```python
from build123d import *

# Parameters (mm, degrees)
SKETCH_1_W                   = 36
SKETCH_1_H                   = 18.5
EXTRUDE_1_DEPTH              = 8
HOLE_WIZARD_M2_1_D           = 2.4
HOLE_WIZARD_M2_1_CBORE_D     = 4.4
HOLE_WIZARD_M2_1_CBORE_DEPTH = 3.5
SKETCH_8_W                   = 60
SKETCH_8_H                   = 30
EXTRUDE_2_DEPTH              = 10
EXTRUDE_3_DEPTH              = 2.5


with BuildPart() as part:
    # 草图1 → 凸台-拉伸1 (new body)
    with BuildSketch(Plane(origin=(0, 0, 0), x_dir=(1, 0, 0), z_dir=(0, 1, 0))):
        with Locations((-18, 0)):
            Rectangle(SKETCH_1_W, SKETCH_1_H)
        Polygon((-6.8, 6.25), (-29.2, 6.25), (-33, 6.25), (-33, -6.25), (-29.2, -6.25), (-6.8, -6.25), align=None, mode=Mode.SUBTRACT)
    extrude(amount=EXTRUDE_1_DEPTH)

    # M2 凹头盖螺钉的柱形沉头孔1 (through all)
    with Locations(Plane(origin=(-4.15, 8, 0), x_dir=(0, 0, 1), z_dir=(0, 1, 0))):
        with Locations((0, 0)):
            CounterBoreHole(HOLE_WIZARD_M2_1_D / 2, HOLE_WIZARD_M2_1_CBORE_D / 2, HOLE_WIZARD_M2_1_CBORE_DEPTH)

    # 草图4 → 放样1 section 0
    with BuildSketch(Plane(origin=(0, 0, 0), x_dir=(0, 0, -1), z_dir=(1, 0, 0))):
        with BuildLine():
            Line((9.25, 8), (-9.25, 8))
            Line((-9.25, 8), (-9.25, 0))
            Line((-9.25, 0), (9.25, 0))
            Line((9.25, 0), (9.25, 8))
        make_face()
    # 草图5 → 放样1 section 1
    with BuildSketch(Plane(origin=(60, 0, 0), x_dir=(0, 0, -1), z_dir=(1, 0, 0))):
        with BuildLine():
            Line((-2.5, 8), (2.5, 8))
            Line((2.5, 8), (2.5, 0))
            Line((2.5, 0), (-2.5, 0))
            Line((-2.5, 0), (-2.5, 8))
        make_face()
    loft()

    # 草图8 → 凸台-拉伸2 (add)
    with BuildSketch(Plane(origin=(60, 0, 0), x_dir=(0, 0, -1), z_dir=(1, 0, 0))):
        with Locations((0, 15)):
            Rectangle(SKETCH_8_W, SKETCH_8_H)
    extrude(amount=-EXTRUDE_2_DEPTH)

    # 草图11 → 凸台-拉伸3 (add, symmetric)
    with BuildSketch(Plane.XY):
        Polygon((50, 28), (20, 8), (50, 8), align=None)
    extrude(amount=EXTRUDE_3_DEPTH, both=True)


solid = part.part
```
The model under review builds one solid part; all positions refer to its coordinate system, in mm. A direction names the side the tool comes from. Coordinates: 2 decimals unless noted, no trailing zeros. Loops run counter-clockwise (first coordinate to the right, second up) from the corner with the lowest first, then second, coordinate; pieces in that order, holes last. Notation, with made-up numbers: (-28, -19) -> (1, -19) arc R18 cw to (1, 5) -> close; hole circle Ø1 at (-17.75, 54.25). An arc over 180 degrees is marked (long way). Answer as CSV lines item,"result".
Item 1: Take a section at A-A, the plane x = -4.15. State the section outline as (y, z) points, and give its area (3 significant figures).
Results below:
outline,"(0, -9.25) -> (8, -9.25) -> (8, -2.2) -> (4.5, -2.2) -> (4.5, -1.2) -> (0, -1.2) -> close; (0, 1.2) -> (4.5, 1.2) -> (4.5, 2.2) -> (8, 2.2) -> (8, 9.25) -> (0, 9.25) -> close"
area,"122 mm2"
Item 2: Take a section at C-C, the plane y = 18.5. State the section outline as (x, z) points, and give its area (3 significant figures).
Results below:
outline,"(35.75, -2.5) -> (50, -2.5) -> (50, -30) -> (60, -30) -> (60, 30) -> (50, 30) -> (50, 2.5) -> (35.75, 2.5) -> close"
area,"671 mm2"
Item 3: Take a section at D-D, the plane z = 11. State the section outline as (x, y) points.
Results below:
outline,"(50, 0) -> (60, 0) -> (60, 30) -> (50, 30) -> close"
Item 4: Insertion check: pin 1 (4 mm diameter, centred on x = -4.15, z = 0, fed in from +Y); pin 2 (6 mm diameter, centred on x = 12.5, y = 6, fed in from -Z); pin 3 (6.5 mm diameter, centred on x = -17, y = 6, fed in from +Z); pin 4 (5 mm diameter, centred on x = -22.5, z = 3, fed in from +Y). Each pin has a flat end and moves straight along its axis. Give the tip position at first contact, or say it passes through.
Results below:
pin 1,"stops at y = 4.5"
pin 2,"stops at z = -8.18"
pin 3,"stops at z = 9.25"
pin 4,"passes through"
Item 5: Draft analysis for pull direction X (two halves, no side actions). For faces 1 (the cylindrical face through (-4.1, 6.3, -2.2)), 2 (the flat face through (55, 15, -30)), 3 (the flat face through (-36, 4, 0)), state which applies: +X half, -X half, draft (parallel to the pull), parting line (faces both ways), or undercut.
Results below:
face 1,"undercut"
face 2,"draft"
face 3,"-X half"
Item 6: For L1, parallel to X at y = 3, z = 0; L2, parallel to X at y = 6, z = 0; L3, parallel to Z at x = -4, y = 2, list the stretches that pass through material, from the lowest coordinate up.
Results below:
L1,"x = -36 to -33, -6.8 to -5.35, -2.95 to 60"
L2,"x = -36 to -33, -6.8 to -6.35, -1.95 to 60"
L3,"z = -9.25 to -1.19, 1.19 to 9.25"
Item 7: Take a section at B-B, the plane z = 0. State the section outline as (x, y) points.
Results below:
outline,"(-36, 0) -> (-33, 0) -> (-33, 8) -> (-36, 8) -> close; (-6.8, 0) -> (-5.35, 0) -> (-5.35, 4.5) -> (-6.35, 4.5) -> (-6.35, 8) -> (-6.8, 8) -> close; (-2.95, 0) -> (60, 0) -> (60, 30) -> (50, 30) -> (50, 28) -> (20, 8) -> (-1.95, 8) -> (-1.95, 4.5) -> (-2.95, 4.5) -> close"
Item 8: Machinability: for faces 4 (the flat face through (41, 14, 2.5)), 5 (the flat face through (25.35, 4.06, 6.4)), 6 (the flat face through (-4.1, 4.5, 1.4)), 7 (the flat face through (25.35, 3.94, -6.4)), 8 (the flat face through (-20, 4, 6.25)), which of the approach directions +Z, -Z, +X, -X, +Y, -Y give a long, thin tool a straight path to every point of the face, cutting with its end or side? Answer none if there is none.
Results below:
face 4,"+Z, -X, +Y"
face 5,"+Z, +Y, -Y"
face 6,"+Y"
face 7,"-Z, +Y, -Y"
face 8,"+Y, -Y"
